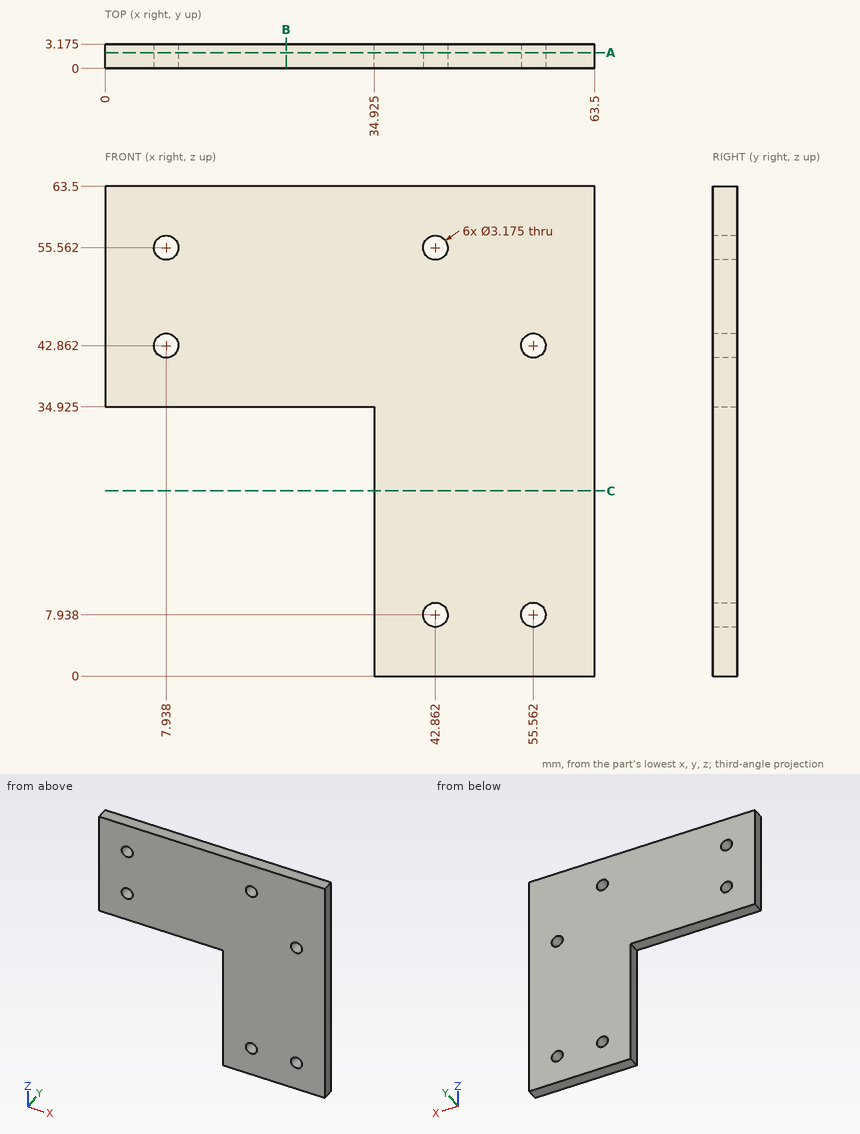
Could you check a few things on this drawing? It's one solid part, dimensions in mm from its lowest x, y, z. Coordinates: 2 decimals unless noted, no trailing zeros. Order: outer loops, then holes, each group sorted by start corner. A loop starts at its lowest first (then second) coordinate and runs counter-clockwise, first axis right, second up. Notation, with made-up numbers: (22, 34) -> (46, 34) arc R23 cw to (46, 58) -> close; hole circle Ø2 at (67, 80). An arc over 180 degrees is marked (long way). One line per item, written item: value. Start each with the question number.
1) Imagine slicing it at A-A on y = 2.05. Count the separate pieces of the cut face and the enclosed holes in it, plus the area to 4 significant figures.
2) If I drill on L1, parallel to X at y = 1.85, z = 55.5; L2, parallel to X at y = 0.2, z = 8 (1 decimal); L3, parallel to X at y = 2.7, z = 20.5 (1 decimal), over which ranges is the centre line in solid material (lowest first)? Write a range as [from, to].
3) I'm going to push flat-ended pins straight in: pin 1 (1.6 mm diameter, centred on x = 14, y = 1, fed in from -Z) (1 decimal); pin 2 (5 mm diameter, centred on x = 55.56, z = 42.86, fed in from -Y); pin 3 (3 mm diameter, centred on x = 7.94, z = 42.86, fed in from -Y). Where does each tip first touch, or does it pass through?
4) Imagine slicing it at B-B on x = 23.5. List the corners of the cut face in (y, z) for me (1 decimal).
5) Imagine slicing it at C-C on z = 24. List the corners of the cut face in (x, y) for me (1 decimal).
Answer list:
1. separate pieces: 1
1. enclosed holes: 6
1. area: 2,765 mm2
2. L1: x = [0, 6.35], [9.52, 41.28], [44.45, 63.5]
2. L2: x = [34.9, 41.3], [44.4, 54], [57.1, 63.5]
2. L3: x = [34.9, 63.5]
3. pin 1: stops at z = 34.9
3. pin 2: stops at y = 0
3. pin 3: passes through
4. outline: (0, 34.9) -> (3.2, 34.9) -> (3.2, 63.5) -> (0, 63.5) -> close
5. outline: (34.9, 0) -> (63.5, 0) -> (63.5, 3.2) -> (34.9, 3.2) -> close
